The model under review builds one solid part; all positions refer to its coordinate system, in mm. Face numbers are marked on the shaded views. Give positions to 0.01 mm unless a question says otherwise; leave off trailing zeros. Write each loop counter-clockwise with the first axis right and the second up, starting at its lowest first coordinate (ties: lowest second). Pieces come first, ordered by that corner, then holes. Notation, with made-up numbers: (-26.5, 46) -> (-0.5, 46) arc R10 cw to (-0.5, 61) -> close; hole circle Ø10 at (46.25, 11). An arc over 180 degrees is marked (long way). Use CSV: the item, a comma, the result in double quotes.
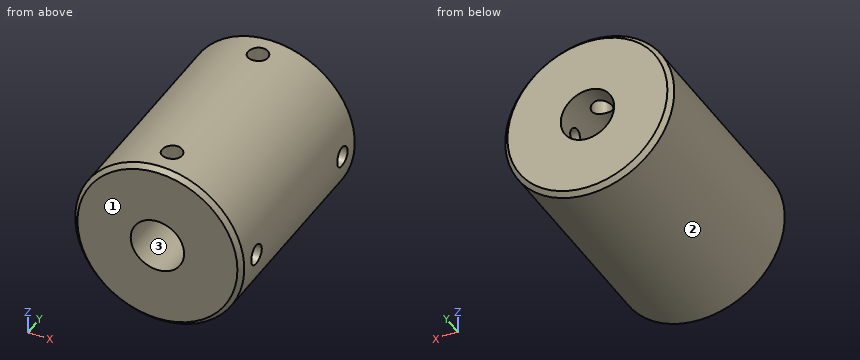
```python
from build123d import *

# Parameters (mm, degrees)
SKETCH1_R                      = 9.5
BOSS_EXTRUDE1_DEPTH            = 25
CHAMFER1_SIZE                  = 0.508
F_6_0MM_DOWEL_HOLE1_D          = 6
SKETCH7_W                      = 1.1303
SKETCH7_H                      = 9.5
F_4_40_TAPPED_HOLE1_AT_2_COUNT = 2
F_4_40_TAPPED_HOLE1_AT_2_PITCH = 18.65
SKETCH10_W                     = 1.1303
SKETCH10_H                     = 9.5
F_4_40_TAPPED_HOLE2_AT_2_COUNT = 2
F_4_40_TAPPED_HOLE2_AT_2_PITCH = 18.65


with BuildPart() as part:
    # Sketch1 → Boss-Extrude1 (new body)
    with BuildSketch(Plane(origin=(0, 0, 0), x_dir=(1, 0, 0), z_dir=(0, 1, 0))):
        with Locations(Location((0, 0, 0), (0, 0, 270))):
            Circle(SKETCH1_R)
    extrude(amount=BOSS_EXTRUDE1_DEPTH)

    # Chamfer1
    chamfer1_edges = [part.edges().sort_by_distance(p)[0] for p in [
        (0, 0, -9.5),
        (0, 25, -9.5),
    ]]
    chamfer(chamfer1_edges, length=CHAMFER1_SIZE)

    # Ø6.0mm Dowel Hole1 (through all)
    with Locations(Plane(origin=(0, 25, 0), x_dir=(1, 0, 0), z_dir=(0, 1, 0))):
        with Locations((0, 0)):
            Hole(F_6_0MM_DOWEL_HOLE1_D / 2)

    # Sketch7 → #4-40 Tapped Hole1 (revolve, cut)
    with BuildSketch(Plane.ZX.offset(21.825)):
        with Locations((0.56515, 4.75)):
            Rectangle(SKETCH7_W, SKETCH7_H)
    f_4_40_tapped_hole1 = revolve(axis=Axis((-6.35, 21.825, 0), (1, 0, 0)), mode=Mode.SUBTRACT)

    # #4-40 Tapped Hole1 at 2: #4-40 Tapped Hole1 ×2
    with Locations(*[(0, -i * F_4_40_TAPPED_HOLE1_AT_2_PITCH, 0) for i in range(1, F_4_40_TAPPED_HOLE1_AT_2_COUNT)]):
        add(f_4_40_tapped_hole1, mode=Mode.SUBTRACT)

    # Sketch10 → #4-40 Tapped Hole2 (revolve, cut)
    with BuildSketch(Plane(origin=(0, 21.825, 0), x_dir=(0, 1, 0), z_dir=(1, 0, 0))):
        with Locations((0.56515, 4.75)):
            Rectangle(SKETCH10_W, SKETCH10_H)
    f_4_40_tapped_hole2 = revolve(axis=Axis((0, 21.825, -6.35), (0, 0, 1)), mode=Mode.SUBTRACT)

    # #4-40 Tapped Hole2 at 2: #4-40 Tapped Hole2 ×2
    with Locations(*[(0, -i * F_4_40_TAPPED_HOLE2_AT_2_PITCH, 0) for i in range(1, F_4_40_TAPPED_HOLE2_AT_2_COUNT)]):
        add(f_4_40_tapped_hole2, mode=Mode.SUBTRACT)


solid = part.part
```
Q1. Consider section A-A (z = 0). Write out the cut boundary in (x, y).
Derived:
outline,"(-9.5, 0.51) -> (-8.99, 0) -> (-3, 0) -> (-3, 25) -> (-8.99, 25) -> (-9.5, 24.49) -> close; (3, 0) -> (8.99, 0) -> (9.5, 0.51) -> (9.5, 2.04) -> (3, 2.04) -> close; (3, 4.31) -> (9.5, 4.31) -> (9.5, 20.69) -> (3, 20.69) -> close; (3, 22.96) -> (9.5, 22.96) -> (9.5, 24.49) -> (8.99, 25) -> (3, 25) -> close"
Q2. To check wall thickness, follow probe 1 along Y at (x, z) = (6.75, 0); probe 2 along X at (y, z) = (20.75, 0.75); probe 3 along Z at (x, y) = (4, 3.5). State the ranges of each line that lie inside material, in increasing order.
Derived:
probe 1,"y = 0 to 2.04, 4.31 to 20.69, 22.96 to 25"
probe 2,"x = -9.47 to -2.9, 2.9 to 9.47"
probe 3,"z = -8.62 to -1.08, 1.08 to 8.62"
Q3. The part is to be moulded in two halves that separate along X. For the marked faces 1, 2 and 3, say which applies: pulls with the +X half, pulls with the -X half, needs draft (parallel to the pull), parting line crosses it, or undercut.
Derived:
face 1,"needs draft"
face 2,"parting line crosses it"
face 3,"undercut"
Q4. Consider section D-D (x = 7.75). State how many separate pieces and enclosed holes the cut face has, then the cut area to 3 significant figures.
Derived:
separate pieces,"1"
enclosed holes,"2"
area,"266 mm2"
Q5. Consider section C-C (y = 16.5). Write out the cut boundary in (x, z).
Derived:
outline,"circle Ø19 at (0, 0); hole circle Ø6 at (0, 0)"
Q6. Insertion check: pin 1 (2 mm diameter, centred on y = 3.175, z = 0, fed in from +X); pin 2 (3 mm diameter, centred on y = 18.5, z = -6, fed in from +X); pin 3 (1.5 mm diameter, centred on x = -3, y = 14.5, fed in from -Z). Each pin has a flat end and moves straight along its axis. Give the tip position at first contact, or say it passes through.
Derived:
pin 1,"stops at x = -2.83"
pin 2,"stops at x = 8.37"
pin 3,"stops at z = -9.23"
Q7. Consider section B-B (x = 0). Write out the cut boundary in (y, z).
Derived:
outline,"(0, -8.99) -> (0.51, -9.5) -> (24.49, -9.5) -> (25, -8.99) -> (25, -3) -> (0, -3) -> close; (0, 3) -> (2.04, 3) -> (2.04, 9.5) -> (0.51, 9.5) -> (0, 8.99) -> close; (4.31, 3) -> (20.69, 3) -> (20.69, 9.5) -> (4.31, 9.5) -> close; (22.96, 3) -> (25, 3) -> (25, 8.99) -> (24.49, 9.5) -> (22.96, 9.5) -> close"
